```python
from build123d import *

# Parameters (mm, degrees)
BASE_FLANGE1_DEPTH       = 1
SKETCHED_START           = 11.616422755
SKETCHED_BEND1_OUTLINE_W = 40
SKETCHED_BEND1_OUTLINE_H = 1
SKETCHED_BEND1_DEPTH     = 28.383577245
SKETCHED_START_2         = 10.821902755
SKETCHED_BEND1_2_DEPTH   = 0.00548
SKETCHED_START_3         = 9.821902755
SKETCHED_BEND1_3_DEPTH   = 2
SKETCHED_START_4         = -20
SKETCHED_BEND1_4_DEPTH   = 40
SKETCH7_R                = 2.025
CUT_EXTRUDE1_DEPTH       = 10
F_6_CLEARANCE_HOLE1_D    = 3.7973
F_4_CLEARANCE_HOLE2_D    = 3.2639


with BuildPart() as part:
    # Base-Flange1: sheet metal written as solids
    # Sketch1 → Base-Flange1 (new body)
    with BuildSketch(Plane(origin=(0, 0, 0), x_dir=(1, 0, 0), z_dir=(0, 1, 0))):
        with BuildLine():
            Line((-20, -8), (-20, -35))
            ThreePointArc((-20, -35), (-18.535533906, -38.535533906), (-15, -40))
            Line((-15, -40), (15, -40))
            ThreePointArc((15, -40), (18.535533906, -38.535533906), (20, -35))
            Line((20, -35), (20, -8))
            Line((20, -8), (26, -8))
            ThreePointArc((26, -8), (27.414213562, -7.414213562), (28, -6))
            Line((28, -6), (28, 6))
            ThreePointArc((28, 6), (27.414213562, 7.414213562), (26, 8))
            Line((26, 8), (20, 8))
            Line((20, 8), (20, 25))
            ThreePointArc((20, 25), (15.606601718, 35.606601718), (5, 40))
            Line((5, 40), (-5, 40))
            ThreePointArc((-5, 40), (-15.606601718, 35.606601718), (-20, 25))
            Line((-20, 25), (-20, 8))
            Line((-20, 8), (-26, 8))
            ThreePointArc((-26, 8), (-27.414213562, 7.414213562), (-28, 6))
            Line((-28, 6), (-28, -6))
            ThreePointArc((-28, -6), (-27.414213562, -7.414213562), (-26, -8))
            Line((-26, -8), (-20, -8))
        make_face()
    extrude(amount=-BASE_FLANGE1_DEPTH)

    # Sketched Bend1: read off the stored shape, not the designer's step
    # Sketched Bend1 outline → Sketched Bend1 (cut)
    with BuildSketch(Plane.XY.offset(SKETCHED_START)):
        with Locations((0, -0.5)):
            Rectangle(SKETCHED_BEND1_OUTLINE_W, SKETCHED_BEND1_OUTLINE_H)
    extrude(amount=SKETCHED_BEND1_DEPTH, mode=Mode.SUBTRACT)

    # Sketched Bend1 2 outline → Sketched Bend1 2 (add)
    with BuildSketch(Plane.XY.offset(SKETCHED_START_2)):
        with BuildLine():
            Line((20, 0), (20, 23.821902755))
            ThreePointArc((20, 23.821902755), (18.535533906, 27.357436661), (15, 28.821902755))
            Line((15, 28.821902755), (-15, 28.821902755))
            ThreePointArc((-15, 28.821902755), (-18.535533906, 27.357436661), (-20, 23.821902755))
            Line((-20, 23.821902755), (-20, 0))
            Line((-20, 0), (20, 0))
        make_face()
    extrude(amount=SKETCHED_BEND1_2_DEPTH)

    # Sketched Bend1 3 outline → Sketched Bend1 3 (add)
    with BuildSketch(Plane.XY.offset(SKETCHED_START_3)):
        with BuildLine():
            Line((20, 0), (20, 23.821902755))
            ThreePointArc((20, 23.821902755), (18.535533906, 27.357436661), (15, 28.821902755))
            Line((15, 28.821902755), (-15, 28.821902755))
            ThreePointArc((-15, 28.821902755), (-18.535533906, 27.357436661), (-20, 23.821902755))
            Line((-20, 23.821902755), (-20, 0))
            Line((-20, 0), (20, 0))
        make_face()
    extrude(amount=SKETCHED_BEND1_3_DEPTH)

    # Sketched Bend1 4 outline → Sketched Bend1 4 (cut)
    with BuildSketch(Plane.YZ.offset(SKETCHED_START_4)):
        with BuildLine():
            Line((28.821902755, 9.821902755), (28.821902755, 10.821902755))
            Line((28.821902755, 10.821902755), (1, 10.821902755))
            ThreePointArc((1, 10.821902755), (0.292893219, 10.529009536), (0, 9.821902755))
            Line((0, 9.821902755), (28.821902755, 9.821902755))
        make_face()
        with BuildLine():
            ThreePointArc((-1, 9.821902755), (-0.414213562, 11.236116317), (1, 11.821902755))
            Line((1, 11.821902755), (0, 11.821902755))
            Line((0, 11.821902755), (0, 11.616422755))
            Line((0, 11.616422755), (-1, 11.616422755))
            Line((-1, 11.616422755), (-1, 9.821902755))
        make_face()
    extrude(amount=SKETCHED_BEND1_4_DEPTH, mode=Mode.SUBTRACT)

    # Sketch7 → Cut-Extrude1 (cut)
    with BuildSketch(Plane(origin=(0, 0, 0), x_dir=(1, 0, 0), z_dir=(0, 1, 0))):
        with Locations(Location((0, 32.178097245, 0), (0, 0, 270))):
            Circle(SKETCH7_R)
    extrude(amount=-CUT_EXTRUDE1_DEPTH, mode=Mode.SUBTRACT)

    # #6 Clearance Hole1 (through all)
    with Locations(Plane(origin=(0, 0, 10.821902755), x_dir=(-1, 0, 0), z_dir=(0, 0, -1))):
        with Locations((13, 13.821902755), (-13, 13.821902755), (0, 23.821902755)):
            Hole(F_6_CLEARANCE_HOLE1_D / 2)

    # #4 Clearance Hole2 (through all)
    with Locations(Plane(origin=(0, 0, 0), x_dir=(1, 0, 0), z_dir=(0, 1, 0))):
        with Locations((-24, 4), (-24, -4), (24, 4), (24, -4), (-12, 32.178097245), (12, 32.178097245)):
            Hole(F_4_CLEARANCE_HOLE2_D / 2)


solid = part.part
```
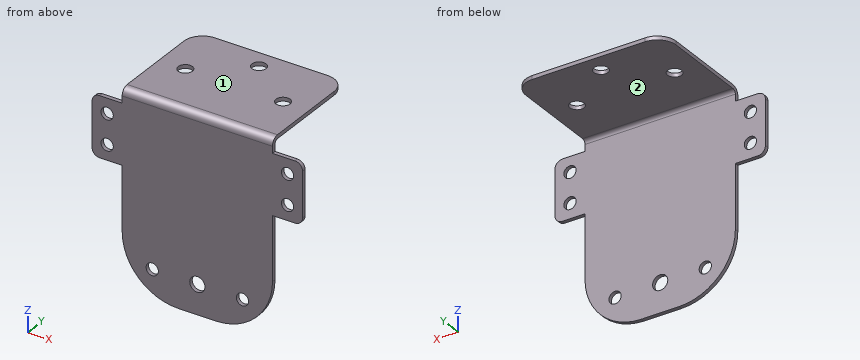
The model under review builds one solid part; all positions refer to its coordinate system, in mm. Face numbers are marked on the shaded views. A direction names the side the tool comes from. Give positions to 0.01 mm unless a question says otherwise; leave off trailing zeros. Loops run counter-clockwise (first coordinate to the right, second up) from the corner with the lowest first, then second, coordinate; pieces in that order, holes last. Notation, with made-up numbers: (83.25, -10.75) -> (99.25, -10.75) arc R27 ccw to (99.25, 12.25) -> close; hole circle Ø8 at (56, 57). An arc over 180 degrees is marked (long way). Use CSV: the item, a comma, the result in double quotes.
1. Consider section D-D, the plane x = -12. Write out the cut boundary in (y, z), then the cut area to 3 significant figures.
Result:
outline,"(-1, -38.27) -> (0, -38.27) -> (0, -33.81) -> (-1, -33.81) -> close; (-1, -30.55) -> (0, -30.55) -> (0, 9.82) arc R1 cw to (1, 10.82) -> (12.21, 10.82) -> (12.21, 11.82) -> (1, 11.82) arc R2 ccw to (-1, 9.82) -> close; (15.44, 10.82) -> (28.82, 10.82) -> (28.82, 11.82) -> (15.44, 11.82) -> close"
area,"71.8 mm²"
2. Consider section A-A, the plane z = 4. Write out the cut boundary in (x, y), then the cut area to 3 significant figures.
Result:
outline,"(-28, -1) -> (-25.63, -1) -> (-25.63, 0) -> (-28, 0) -> close; (-22.37, -1) -> (22.37, -1) -> (22.37, 0) -> (-22.37, 0) -> close; (25.63, -1) -> (28, -1) -> (28, 0) -> (25.63, 0) -> close"
area,"49.5 mm²"
3. For P1, Ø1.5, axis at x = 6, y = 16.5, coming from the -Z side; P2, Ø10, axis at x = -8, z = -10.5, coming from the +Y side; P3, Ø0.8, axis at x = -22.5, y = -0.5, coming from the -Z side, all flat-tipped, find the tip position at first contact; note any pin that passes through.
Result:
P1,"stops at z = 10.82"
P2,"stops at y = 0"
P3,"stops at z = -8"
4. Consider section C-C, the plane y = 15. Write out the cut boundary in (x, z).
Result:
outline,"(-20, 10.82) -> (-14.49, 10.82) -> (-14.49, 11.82) -> (-20, 11.82) -> close; (-11.51, 10.82) -> (11.51, 10.82) -> (11.51, 11.82) -> (-11.51, 11.82) -> close; (14.49, 10.82) -> (20, 10.82) -> (20, 11.82) -> (14.49, 11.82) -> close"
5. To check wall thickness, follow probe 1 along Z at (x, y) = (-24, -0.8); probe 2 along Z at (x, y) = (10.5, 18.5); probe 3 along Y at (x, z) = (11, -2.5). State the ranges of each line that lie inside material, in increasing order. Write a range as from..to.
Result:
probe 1,"z = -8..-5.63, -2.37..2.37, 5.63..8"
probe 2,"z = 10.82..11.82"
probe 3,"y = -1..0"
6. Machinability: for the marked faces 1 and 2, which of the approach directions +Z, -Z, +X, -X, +Y, -Y give a long, thin tool a straight path to every point of the face, cutting with its end or side? Answer none if there is none.
Result:
face 1,"+Z, +X, -X, +Y, -Y"
face 2,"-Z, +X, -X, +Y"
7. Consider section B-B, the plane x = 0. Write out the cut boundary in (y, z), then the cut area to 3 significant figures.
Result:
outline,"(-1, -40) -> (0, -40) -> (0, -34.2) -> (-1, -34.2) -> close; (-1, -30.15) -> (0, -30.15) -> (0, 9.82) arc R1 cw to (1, 10.82) -> (21.92, 10.82) -> (21.92, 11.82) -> (1, 11.82) arc R2 ccw to (-1, 9.82) -> close; (25.72, 10.82) -> (28.82, 10.82) -> (28.82, 11.82) -> (25.72, 11.82) -> close"
area,"72.2 mm²"
